Verification items for this drawing (mm, ordinates from the low corner). A direction names the side the tool comes from. Round coordinates to 2 decimals unless told otherwise and drop trailing zeros. One line per question, with ' | ' between items. Start each with the question number.
Q1. Material ranges on line 1 along Y through (x, z) = (2, 12); line 2 along Z through (x, y) = (40, 70.5); line 3 along X through (y, z) = (47, 11), recorded low to high.
Q2. Sectioned sample at A-A, the plane z = 12.7. Give the number of separate pieces and of enclosed holes in the cut face, then the cut area to 3 significant figures.
Q3. Gauge pin test, flat ends, axial feed: P1, Ø17, axis at x = 25.5, y = 46, coming from the -Z side; P2, Ø8.5, axis at y = 76.2, z = 12.7, coming from the +X side. Record the tip position at first contact, or that the pin passes through.
Q4. Tool access check on the marked faces 1 and 2. Record the directions out of +Z, -Z, +X, -X, +Y, -Y that give a thin tool (end or side, any length) a straight path to the whole face; none if there is none.
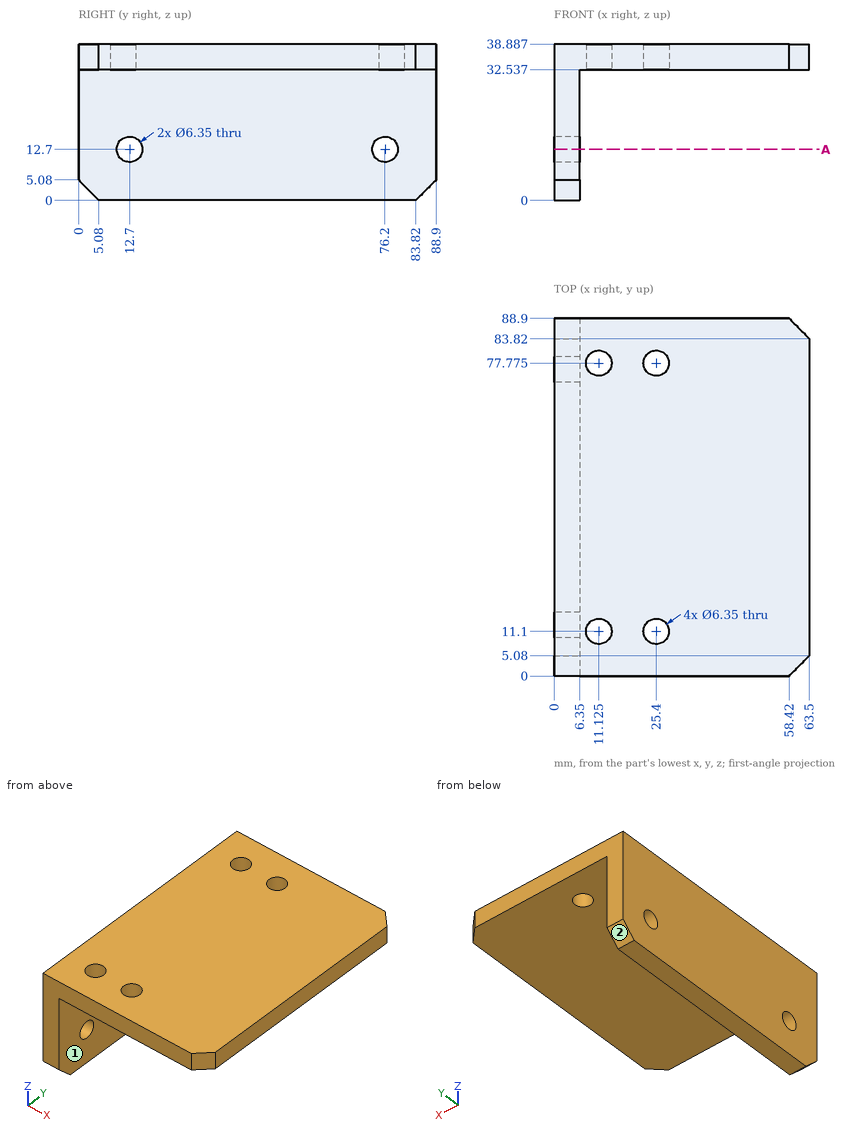
Determined:
1) line 1: y = 0 to 9.6, 15.8 to 73.1, 79.3 to 88.9 | line 2: z = 32.54 to 38.89 | line 3: x = 0 to 6.35
2) separate pieces: 3 | enclosed holes: 0 | area: 484 mm2
3) P1: stops at z = 32.54 | P2: stops at x = 6.35
4) face 1: -Z, +X, +Y, -Y | face 2: -Z, +X, -X, +Y
